Could you check a few things on this model? Use its own coordinates, in mm. Face numbers are marked on the shaded views. A direction names the side the tool comes from. Give positions to 0.01 mm unless a question says otherwise; leave off trailing zeros. Loops run counter-clockwise (first coordinate to the right, second up) from the corner with the lowest first, then second, coordinate; pieces in that order, holes last. Notation, with made-up numbers: (35.5, -26) -> (53.5, -26) arc R22 ccw to (53.5, -20) -> close; hole circle Ø6 at (-23.75, 54). An arc over 180 degrees is marked (long way). Write item = value, one per line. Start each with the question number.
1) On a 3-axis mill with a long thin cutter (end or side, diameter ignored), from which of +Z, -Z, +X, -X, +Y, -Y can I reach the whole of each face in a straight line? I mean the marked faces 1, 2 and 3. Say none if no direction works.
2) I want a section at A-A (x = 0). List the corners of the cut face in (y, z) for me, and give its area (4 significant figures).
3) I want a section at C-C (z = 7.25). List the corners of the cut face in (x, y) for me.
4) I need wall thicknesses on probe 1 along Z at (x, y) = (0, 6); probe 2 along Z at (x, y) = (0, -5); probe 3 along Z at (x, y) = (1.5, 3). Which ranges of each line are inside material? Lowest first, please. Write a range as from..to.
5) I want a section at B-B (y = 5). List the corners of the cut face in (x, z) for me.
6) I'm going to push flat-ended pins straight in: pin 1 Ø1 at (y, z) = (-9.5, 8.5) entering from +X; pin 2 Ø3 at (x, y) = (1.5, -2.5) entering from +Z. Where does each tip first touch, or does it pass through?
7) If we mould it in two halves opening along X, with no side actions, what happens to the marked faces 4, 5 and 6? For each: +X half, -X half, draft (parallel to the pull), parting line (faces both ways), or undercut.
8) I want a section at D-D (x = -4). List the corners of the cut face in (y, z) for me, and give its area (3 significant figures).
Autodesk Fusion 360 part; units mm, degrees
sketch "Sketch1" plane through (0, 0, 0) normal (0, 1, 0) x (1, 0, 0)
  line L0 (-7.5, 6.25) -> (7.5, 6.25)
  line L1 (7.5, 6.25) -> (7.5, -6.25)
  line L2 (-7.5, -6.25) -> (-7.5, 6.25)
  line L3 (-7.5, 6.25) -> (7.5, -6.25) construction
  line L4 (7.5, 6.25) -> (-7.5, -6.25) construction
  line L5 (7.5, -6.25) -> (6, -6.25)
  line L6 (-6, -6.25) -> (-7.5, -6.25)
  arc A0 (-6, -6.25) -> (6, -6.25) centre (0, -6.25) ccw
  arc A1 (0.3096, -0.258) -> (-0.3096, -0.258) centre (0, -6.25) ccw
  dimension "d1" = 15
  dimension "d2" = 12.5
  dimension "d3" = 12
extrude "Extrude1" add sketch "Sketch1" along normal blind 20
sketch "Sketch2" plane through (0, 0, 0) normal (0, -1, 0) x (1, 0, 0)
  line L0 (-6, 6.25) -> (-7.5, 6.25)
  line L1 (-7.5, 6.25) -> (-7.5, -6.25)
  line L2 (-7.5, -6.25) -> (7.5, -6.25)
  line L3 (7.5, -6.25) -> (7.5, 6.25)
  line L4 (7.5, 6.25) -> (6, 6.25)
  arc A0 (6, 6.25) -> (-6, 6.25) centre (0, 6.25) ccw
  line L5 (4.75, -3.5) -> (-4.75, -3.5)
  line L6 (-4.75, -3.5) -> (-4.75, 3.5)
  line L7 (-4.75, 3.5) -> (4.75, 3.5)
  line L8 (4.75, 3.5) -> (4.75, -3.5)
  line L9 (4.75, -3.5) -> (-4.75, 3.5) construction
  line L10 (-4.75, -3.5) -> (4.75, 3.5) construction
  dimension "d6" = 9.5
  dimension "d7" = 7
extrude "Extrude2" cut sketch "Sketch2" against normal blind 39 contours L5 L6 L7 L8
sketch "Sketch3" plane through (0, 0, 0) normal (0, -1, 0) x (1, 0, 0)
  line L0 (-4.75, -3.5) -> (-4.75, 3.5)
  line L1 (-4.75, 3.5) -> (4.75, 3.5)
  line L2 (4.75, 3.5) -> (4.75, -3.5)
  line L3 (4.75, -3.5) -> (-4.75, -3.5)
  line L4 (-6, 6.25) -> (-7.5, 6.25)
  line L5 (-7.5, 6.25) -> (-7.5, -6.25)
  line L6 (-7.5, -6.25) -> (7.5, -6.25)
  line L7 (7.5, -6.25) -> (7.5, 6.25)
  line L8 (7.5, 6.25) -> (6, 6.25)
  arc A0 (6, 6.25) -> (-6, 6.25) centre (0, 6.25) ccw
  circle A1 centre (0, 6.25) radius 2
  dimension "d10" = 4
extrude "Extrude3" cut sketch "Sketch3" against normal blind 30 contours A1
sketch "Sketch4" plane through (0, 0, 0) normal (0, -1, 0) x (1, 0, 0)
  circle A0 centre (0, 6.25) radius 2
  line L0 (-4.75, -3.5) -> (-4.75, 3.5)
  line L1 (-4.75, 3.5) -> (4.75, 3.5)
  line L2 (4.75, 3.5) -> (4.75, -3.5)
  line L3 (4.75, -3.5) -> (-4.75, -3.5)
  line L4 (-6, 6.25) -> (-7.5, 6.25)
  line L5 (-7.5, 6.25) -> (-7.5, -6.25)
  line L6 (-7.5, -6.25) -> (7.5, -6.25)
  line L7 (7.5, -6.25) -> (7.5, 6.25)
  line L8 (7.5, 6.25) -> (6, 6.25)
  arc A1 (6, 6.25) -> (-6, 6.25) centre (0, 6.25) ccw
  circle A2 centre (0, 6.25) radius 2.35
  dimension "d13" = 0.35
extrude "Extrude4" add sketch "Sketch4" along normal blind 15 contours A2
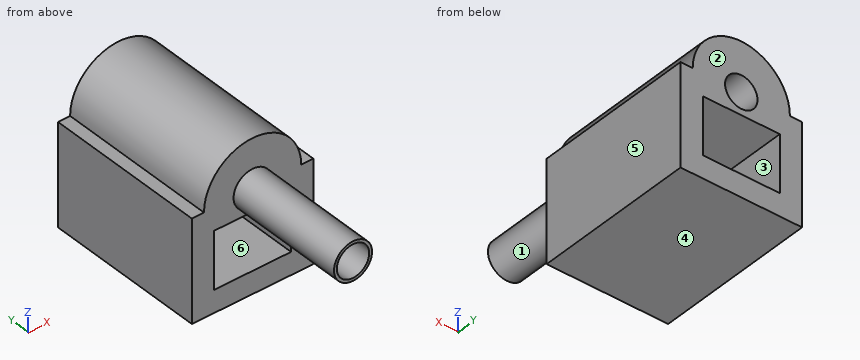
Answer list:
q1.face_1 = -Y
q1.face_2 = +Z, -Z, +X, -X, +Y
q1.face_3 = +Y, -Y
q2.outline = (-15, 3.9) -> (0, 3.9) -> (0, 3.5) -> (20, 3.5) -> (20, 4.25) -> (-15, 4.25) -> close; (-15, 8.25) -> (20, 8.25) -> (20, 12.25) -> (0, 12.25) -> (0, 8.6) -> (-15, 8.6) -> close; (0, -6.25) -> (20, -6.25) -> (20, -3.5) -> (0, -3.5) -> close
q2.area = 160.5 mm^2
q3.outline = (-5.92, 0) -> (-2.13, 0) -> (-2.13, -15) -> (-1.73, -15) -> (-1.73, 20) -> (-5.92, 20) -> close; (1.73, -15) -> (2.13, -15) -> (2.13, 0) -> (5.92, 0) -> (5.92, 20) -> (1.73, 20) -> close
q4.probe_1 = -6.25..-3.5, 3.5..4.25, 8.25..12.25
q4.probe_2 = 3.9..4.25, 8.25..8.6
q4.probe_3 = -6.25..-3.5, 3.5..4.93, 7.57..12.06
q5.outline = (-7.5, -6.25) -> (7.5, -6.25) -> (7.5, 6.25) -> (6, 6.25) arc R6 ccw to (-6, 6.25) -> (-7.5, 6.25) -> close; hole (-4.75, -3.5) -> (4.75, -3.5) -> (4.75, 3.5) -> (-4.75, 3.5) -> close; hole circle Ø4 at (0, 6.25)
q6.pin_1 = 1.57
q6.pin_2 = 8.6
q7.face_4 = draft
q7.face_5 = +X half
q7.face_6 = undercut
q8.outline = (0, -6.25) -> (20, -6.25) -> (20, -3.5) -> (0, -3.5) -> close; (0, 3.5) -> (20, 3.5) -> (20, 10.72) -> (0, 10.72) -> close
q8.area = 199 mm^2
